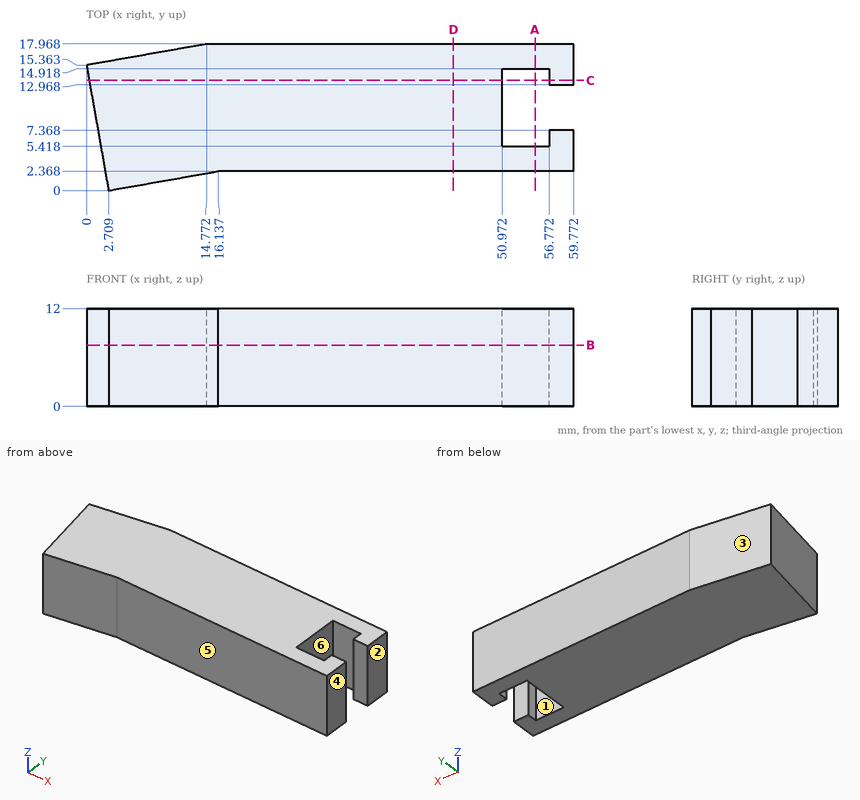
Can you work these out from the drawing? Everything is in mm from the part's minimum corner. A direction names the side the tool comes from. Give positions to 0.01 mm unless a question says otherwise; leave off trailing zeros. Loops run counter-clockwise (first coordinate to the right, second up) from the corner with the lowest first, then second, coordinate; pieces in that order, holes last. Notation, with made-up numbers: (52.5, -11) -> (99.5, -11) arc R21 cw to (99.5, 1) -> close; hole circle Ø3 at (62, 23.5). An arc over 180 degrees is marked (long way). Put each result on its own line as item: value.
(1) I'm going to push flat-ended pins straight in: pin 1 Ø1.5 at (x, y) = (8, 12.5) entering from -Z; pin 2 Ø1 at (x, z) = (43.5, 6) entering from -Y; pin 3 Ø1 at (y, z) = (7, 8.5) entering from -X; pin 4 Ø1 at (y, z) = (14, 3.5) entering from -X. Where does each tip first touch, or does it pass through?
Computed:
pin 1: z = 0
pin 2: y = 2.37
pin 3: x = 1.39
pin 4: x = 0.15
(2) Imagine slicing it at D-D on x = 45. Write out the boundary of the cut face in (y, z), plus the area to 3 significant figures.
Computed:
outline: (2.37, 0) -> (17.97, 0) -> (17.97, 12) -> (2.37, 12) -> close
area: 187 mm^2
(3) Thinking about a two-plate mould opening in X: for the marked faces 1, 2 and 3, which applies, pulls with the +X half, pulls with the -X half, needs draft (parallel to the pull), parting line crosses it, or undercut?
Computed:
face 1: undercut
face 2: pulls with the +X half
face 3: pulls with the -X half
(4) Please list where these lines run through material, in increasing order: probe 1 along Y at (x, z) = (57, 1); probe 2 along Y at (x, z) = (43.5, 4); probe 3 along Y at (x, z) = (56, 8.75). Write a range as [from, to].
Computed:
probe 1: [2.37, 7.37], [12.97, 17.97]
probe 2: [2.37, 17.97]
probe 3: [2.37, 5.42], [14.92, 17.97]
(5) Imagine slicing it at A-A on x = 55. Write out the boundary of the cut face in (y, z).
Computed:
outline: (2.37, 0) -> (5.42, 0) -> (5.42, 12) -> (2.37, 12) -> close; (14.92, 0) -> (17.97, 0) -> (17.97, 12) -> (14.92, 12) -> close
(6) Imagine slicing it at B-B on z = 7.5. Write out the boundary of the cut face in (x, y), plus the area to 3 significant figures.
Computed:
outline: (0, 15.36) -> (2.71, 0) -> (16.14, 2.37) -> (59.77, 2.37) -> (59.77, 7.37) -> (56.77, 7.37) -> (56.77, 5.42) -> (50.97, 5.42) -> (50.97, 14.92) -> (56.77, 14.92) -> (56.77, 12.97) -> (59.77, 12.97) -> (59.77, 17.97) -> (14.77, 17.97) -> close
area: 843 mm^2
(7) Imagine slicing it at C-C on y = 13.5. Write out the boundary of the cut face in (x, z).
Computed:
outline: (0.33, 0) -> (50.97, 0) -> (50.97, 12) -> (0.33, 12) -> close; (56.77, 0) -> (59.77, 0) -> (59.77, 12) -> (56.77, 12) -> close
(8) For the marked faces 4, 5 and 6, which set-ups out of +Z, -Z, +X, -X, +Y, -Y let a thin tool reach every point of the face, with its end or its side?
Computed:
face 4: +Z, -Z, +X, +Y, -Y
face 5: +Z, -Z, +X, -Y
face 6: +Z, -Z
